Check sheet for the modelled part. Datum: model origin and axes. Units: mm. A direction names the side the tool comes from. Coordinates: 2 decimals unless noted, no trailing zeros. Order: outer loops, then holes, each group sorted by start corner. A loop starts at its lowest first (then second) coordinate and runs counter-clockwise, first axis right, second up.
from build123d import *

# Parameters (mm, degrees)
TUBO_RECTANGULAR_60X40X4_DEPTH = 178.5
CORTAR_EXTRUIR1_DEPTH          = 186.370574795


with BuildPart() as part:
    # Sketch1 → Tubo rectangular 60X40X4 (new body)
    with BuildSketch(Plane.YZ):
        with BuildLine():
            Line((-15.5, -30), (15.5, -30))
            ThreePointArc((15.5, -30), (18.681980515, -28.681980515), (20, -25.5))
            Line((20, -25.5), (20, 25.5))
            ThreePointArc((20, 25.5), (18.681980515, 28.681980515), (15.5, 30))
            Line((15.5, 30), (-15.5, 30))
            ThreePointArc((-15.5, 30), (-18.681980515, 28.681980515), (-20, 25.5))
            Line((-20, 25.5), (-20, -25.5))
            ThreePointArc((-20, -25.5), (-18.681980515, -28.681980515), (-15.5, -30))
        make_face()
        with BuildLine():
            Line((-15.5, -26), (15.5, -26))
            ThreePointArc((15.5, -26), (15.853553391, -25.853553391), (16, -25.5))
            Line((16, -25.5), (16, 25.5))
            ThreePointArc((16, 25.5), (15.853553391, 25.853553391), (15.5, 26))
            Line((15.5, 26), (-15.5, 26))
            ThreePointArc((-15.5, 26), (-15.853553391, 25.853553391), (-16, 25.5))
            Line((-16, 25.5), (-16, -25.5))
            ThreePointArc((-16, -25.5), (-15.853553391, -25.853553391), (-15.5, -26))
        make_face(mode=Mode.SUBTRACT)
    extrude(amount=TUBO_RECTANGULAR_60X40X4_DEPTH)

    # Croquis4 → Cortar-Extruir1 (cut, through all)
    with BuildSketch(Plane(origin=(0, 20, 0), x_dir=(1, 0, 0), z_dir=(0, 1, 0))):
        Polygon((0, -30), (2.4, 30), (0, 30), align=None)
    extrude(amount=-CORTAR_EXTRUIR1_DEPTH, mode=Mode.SUBTRACT)


solid = part.part
(1) Cross-section at C-C (y = -6). Enter the section's corners in (x, z).
Filled in:
outline: (0, 30) - (0.16, 26) - (178.5, 26) - (178.5, 30) - close; (2.24, -26) - (2.4, -30) - (178.5, -30) - (178.5, -26) - close
(2) Cross-section at A-A (z = -2.5). Enter the section's corners in (x, y), and give its area (3 significant figures).
Filled in:
outline: (1.3, -20) - (178.5, -20) - (178.5, -16) - (1.3, -16) - close; (1.3, 16) - (178.5, 16) - (178.5, 20) - (1.3, 20) - close
area: 1,420 mm2
(3) Release check for a two-part mould opening along Y. For faces 1 (the flat face through (89, 0, -30)), 2 (the cylindrical face through (88, -18.647, 28.717)), 3 (the flat face through (88, 16, 0)) record: +Y half, -Y half, draft (parallel to the pull), parting line (faces both ways), or undercut.
Filled in:
face 1: draft
face 2: -Y half
face 3: undercut
(4) Cross-section at B-B (x = 87). Enter the section's corners in (y, z).
Filled in:
outline: (-20, -25.5) arc R4.5 ccw to (-15.5, -30) - (15.5, -30) arc R4.5 ccw to (20, -25.5) - (20, 25.5) arc R4.5 ccw to (15.5, 30) - (-15.5, 30) arc R4.5 ccw to (-20, 25.5) - close; hole (-16, -25.5) arc R0.5 ccw to (-15.5, -26) - (15.5, -26) arc R0.5 ccw to (16, -25.5) - (16, 25.5) arc R0.5 ccw to (15.5, 26) - (-15.5, 26) arc R0.5 ccw to (-16, 25.5) - close
(5) Tool access check on faces 4 (the flat face through (1.183, -17.498, 0.42)), 5 (the flat face through (88, 0, 26)). Record the directions out of +Z, -Z, +X, -X, +Y, -Y that give a thin tool (end or side, any length) a straight path to the whole face; none if there is none.
Filled in:
face 4: -Z, -X, +Y, -Y
face 5: +X, -X
(6) Thickness scan on probe 1 along Y at (x, z) = (142, -6); probe 2 along Z at (x, y) = (122.5, 9.5); probe 3 along X at (y, z) = (18, 25.5). Record the ranges inside material, lowest first.
Filled in:
probe 1: y = -20 to -16, 16 to 20
probe 2: z = -30 to -26, 26 to 30
probe 3: x = 0.18 to 178.5
